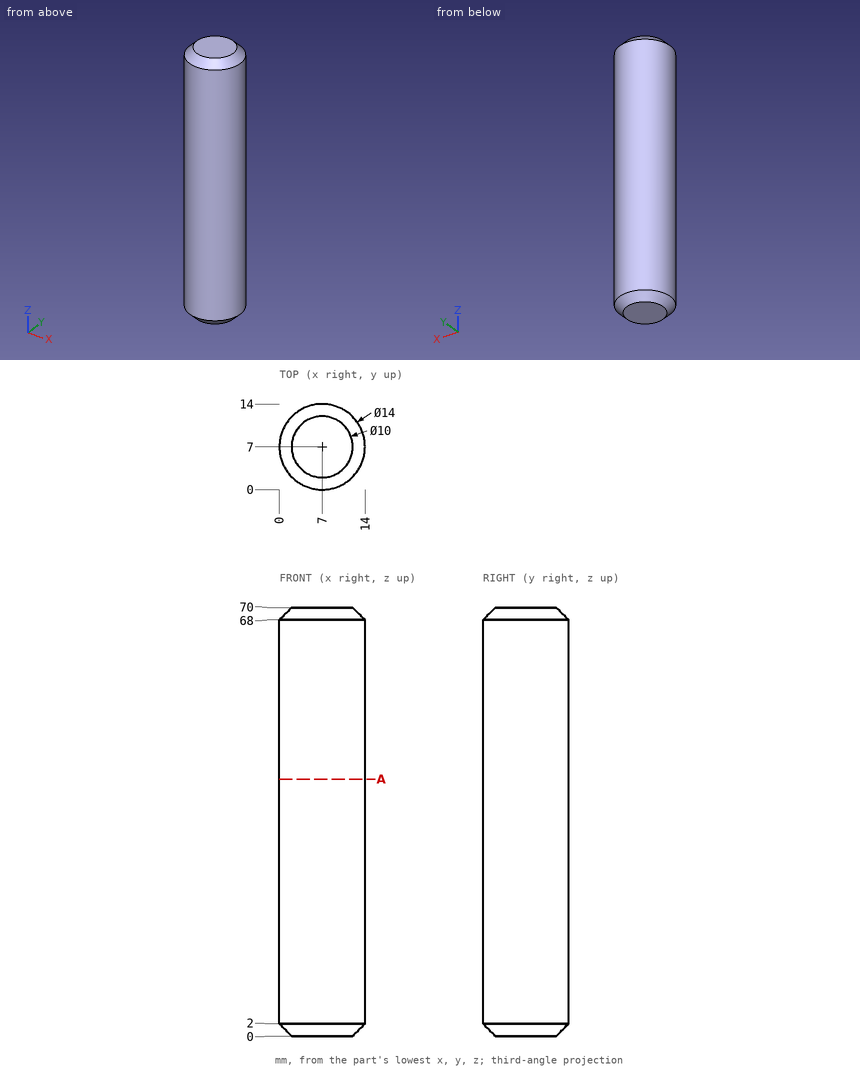
Check sheet for the drawn part. Datum: minimum x, y, z corner. Units: mm. Give positions to 0.01 mm unless a question says otherwise; leave off trailing zeros. Order: outer loops, then holes, each group sorted by start corner. A loop starts at its lowest first (then second) coordinate and runs counter-clockwise, first axis right, second up. Notation, with made-up numbers: (-13.5, -4.5) -> (2.5, -4.5) arc R17 ccw to (2.5, 11.5) -> close; hole circle Ø3 at (60, 57.25). An arc over 180 degrees is marked (long way). One line per item, written item: value.
(1) Gauge pin test, flat ends, axial feed: pin 1 (2 mm diameter, centred on y = 11, z = 24.5, fed in from -X); pin 2 (1 mm diameter, centred on y = 5.5, z = 59, fed in from -X); pin 3 (6 mm diameter, centred on x = 3, z = 37.5, fed in from -Y). Record the tip position at first contact, or that the pin passes through.
Final values:
pin 1: x = 0.68
pin 2: x = 0.07
pin 3: y = 0.07
(2) Sectioned sample at A-A on z = 42. Record the cut outline in (x, y), then the cut area to 3 significant figures.
Final values:
outline: circle Ø14 at (7, 7)
area: 154 mm^2
(3) Scan lines: line 1 along Z through (x, y) = (8.5, 1.5); line 2 along Y through (x, z) = (10, 3); line 3 along Z through (x, y) = (12, 3.75). Record each from-to range of solid material in increasing order. Write a range as [from, to].
Final values:
line 1: [0.7, 69.3]
line 2: [0.68, 13.32]
line 3: [0.96, 69.04]
